Design review of the part built by this model. Coordinates are the model's own, in mm. A direction names the side the tool comes from. Coordinates: 2 decimals unless noted, no trailing zeros. Write each loop counter-clockwise with the first axis right and the second up, starting at its lowest first coordinate (ties: lowest second). Pieces come first, ordered by that corner, then holes.
Q1. For pin 1 Ø2 at (x, y) = (-1, -11.5) entering from +Z; pin 2 Ø1 at (y, z) = (0, -1) entering from +X (3 decimals); pin 3 Ø1.6 at (x, z) = (3.5, -1) entering from -Y, all flat-tipped, find the tip position at first contact; note any pin that passes through.
Q2. Take a section at C-C, the plane z = 12. Write out the cut boundary in (x, y).
Q3. For faces 1 (the cylindrical face through (48.75, -30.82, 0.99)), 2 (the flat face through (56, -1, 7)), 3 (the flat face through (0, -1, 0)), 4 (the flat face through (-1, -34.2, 8)), 5 (the flat face through (35, -1, 0)), list the 3-axis set-ups (+Z, -Z, +X, -X, +Y, -Y) from which the entire face can be reached by the end or side of a thin tool; tool diameter is ignored.
Q4. For L1, parallel to Y at x = 50.25, z = 0.9; L2, parallel to X at y = 30.75, z = 0.55; L3, parallel to X at y = -33, z = 8, list the stretches that pass through material, from the lowest coordinate up.
Q5. The part is to be moulded in two halves that separate along X. For faces 6 (the flat face through (-39, -1, 0)), 7 (the flat face through (-56, -1, 7)), 8 (the flat face through (53.5, 0, 8)), say which applies: released by +X, released by -X, zero draft, split by the parting line, or undercut.
Q6. Take a section at B-B, the plane x = 50.25. Write out the cut boundary in (y, z), plus the area to 3 significant figures.
Q7. Take a section at A-A, the plane y = 11.5. Write out the cut boundary in (x, z) (3 decimals), plus the area to 3 significant figures.
Q8. Take a section at D-D, the plane y = -30.75. Write out the cut boundary in (x, z) (3 decimals), plus the area to 3 significant figures.
from build123d import *

# Parameters (mm, degrees)
SKETCH_W        = 112
SKETCH_H        = 73.4
SKETCH_W_2      = 107
SKETCH_H_2      = 68.4
PAD_DEPTH       = 15
SKETCH001_W     = 6.5
SKETCH001_H     = 6.5
SKETCH001_W_2   = 7.5
PAD001_DEPTH    = 2
SKETCH002_R     = 1.5
POCKET_DEPTH    = 2
SKETCH003_W     = 2
SKETCH003_H     = 73.4
PAD002_DEPTH    = 2
PAD003_DEPTH    = 2
SKETCH005_W     = 15
SKETCH005_H     = 35
POCKET001_DEPTH = 5
SKETCH006_W     = 38.41
SKETCH006_H     = 2
PAD004_DEPTH    = 2


with BuildPart() as part:
    # Sketch → Pad (new body)
    with BuildSketch(Plane.XY):
        Rectangle(SKETCH_W, SKETCH_H)
        Rectangle(SKETCH_W_2, SKETCH_H_2, mode=Mode.SUBTRACT)
    extrude(amount=PAD_DEPTH)

    # Sketch001 (on Face9 of Pad) → Pad001 (join)
    with BuildSketch(Plane(origin=(0, 0, 0), x_dir=(1, 0, 0), z_dir=(0, 0, -1))):
        with Locations((-50.25, 30.95)):
            Rectangle(SKETCH001_W, SKETCH001_H)
        with Locations((-49.75, -30.95)):
            Rectangle(SKETCH001_W_2, SKETCH001_H)
        with Locations((50.25, 30.95)):
            Rectangle(SKETCH001_W, SKETCH001_H)
        with Locations((50.25, -30.95)):
            Rectangle(SKETCH001_W, SKETCH001_H)
    extrude(amount=-PAD001_DEPTH)

    # Sketch002 (on Face22 of Pad001) → Pocket (cut)
    with BuildSketch(Plane(origin=(0, 0, 0), x_dir=(1, 0, 0), z_dir=(0, 0, -1))):
        with Locations((-50.25, 30.75)):
            Circle(SKETCH002_R)
        with Locations((50.25, -30.75)):
            Circle(SKETCH002_R)
        with Locations((-49.75, -30.75)):
            Circle(SKETCH002_R)
        with Locations((50.25, 30.75)):
            Circle(SKETCH002_R)
    extrude(amount=-POCKET_DEPTH, mode=Mode.SUBTRACT)

    # Sketch003 (on Face9 of Pad) → Pad002 (join)
    with BuildSketch(Plane(origin=(0, 0, 0), x_dir=(1, 0, 0), z_dir=(0, 0, -1))):
        with Locations((-20.205, 0)):
            Rectangle(SKETCH003_W, SKETCH003_H)
        with Locations((20.205, 0)):
            Rectangle(SKETCH003_W, SKETCH003_H)
    extrude(amount=PAD002_DEPTH)

    # Sketch004 (on Face4 of Pocket) → Pad003 (join)
    with BuildSketch(Plane(origin=(0, 0, 0), x_dir=(1, 0, 0), z_dir=(0, 0, -1))):
        Polygon((47, -34.2), (-46, -34.2), (-46, -27.7), (-53.5, -27.7), (-53.5, 27.7), (-47, 27.7), (-47, 34.2), (47, 34.2), (47, 27.7), (53.5, 27.7), (53.5, -27.7), (47, -27.7), align=None)
    extrude(amount=-PAD003_DEPTH)

    # Sketch005 (on Face23 of Pad003) → Pocket001 (cut)
    with BuildSketch(Plane.XY.offset(2)):
        with Locations((46, 0)):
            Rectangle(SKETCH005_W, SKETCH005_H)
    extrude(amount=-POCKET001_DEPTH, mode=Mode.SUBTRACT)

    # Sketch006 (on Face11 of Pocket001) → Pad004 (join)
    with BuildSketch(Plane(origin=(0, 0, 0), x_dir=(1, 0, 0), z_dir=(0, 0, -1))):
        with Locations((0, -35.7)):
            Rectangle(SKETCH006_W, SKETCH006_H)
    extrude(amount=PAD004_DEPTH)


solid = part.part
Responses:
1. pin 1: stops at z = 2
1. pin 2: stops at x = 21.205
1. pin 3: stops at y = 34.7
2. outline: (-56, -36.7) - (56, -36.7) - (56, 36.7) - (-56, 36.7) - close; hole (-53.5, -34.2) - (53.5, -34.2) - (53.5, 34.2) - (-53.5, 34.2) - close
3. face 1: +Z, -Z
3. face 2: +Z, -Z, +X, +Y, -Y
3. face 3: -Z, -Y
3. face 4: +Z
3. face 5: -Z, +X, +Y, -Y
4. L1: y = -36.7 to -32.25, -29.25 to -17.5, 17.5 to 29.25, 32.25 to 36.7
4. L2: x = -56 to -51.25, -48.25 to 48.75, 51.75 to 56
4. L3: x = -56 to -53.5, 53.5 to 56
5. face 6: zero draft
5. face 7: released by -X
5. face 8: undercut
6. outline: (-36.7, 0) - (-32.25, 0) - (-32.25, 2) - (-34.2, 2) - (-34.2, 15) - (-36.7, 15) - close; (-29.25, 0) - (-17.5, 0) - (-17.5, 2) - (-29.25, 2) - close; (17.5, 0) - (29.25, 0) - (29.25, 2) - (17.5, 2) - close; (32.25, 0) - (36.7, 0) - (36.7, 15) - (34.2, 15) - (34.2, 2) - (32.25, 2) - close
6. area: 130 mm2
7. outline: (-56, 0) - (-21.205, 0) - (-21.205, -2) - (-19.205, -2) - (-19.205, 0) - (19.205, 0) - (19.205, -2) - (21.205, -2) - (21.205, 0) - (38.5, 0) - (38.5, 2) - (-53.5, 2) - (-53.5, 15) - (-56, 15) - close; (53.5, 0) - (56, 0) - (56, 15) - (53.5, 15) - close
7. area: 267 mm2
8. outline: (-56, 0) - (-51.75, 0) - (-51.75, 2) - (-53.5, 2) - (-53.5, 15) - (-56, 15) - close; (-48.75, 0) - (-21.205, 0) - (-21.205, -2) - (-19.205, -2) - (-19.205, 0) - (19.205, 0) - (19.205, -2) - (21.205, -2) - (21.205, 0) - (48.75, 0) - (48.75, 2) - (-48.75, 2) - close; (51.75, 0) - (56, 0) - (56, 15) - (53.5, 15) - (53.5, 2) - (51.75, 2) - close
8. area: 285 mm2
